Geometry: final body of the model. Coordinates: model frame, mm. Face numbers are marked on the shaded views. Give positions to 0.01 mm unless a question says otherwise; leave off trailing zeros. Order: outer loops, then holes, each group sorted by start corner. A loop starts at its lowest first (then second) coordinate and runs counter-clockwise, first axis right, second up. Notation, with made-up numbers: (-39.5, -10) - (2.5, -10) arc R30 cw to (2.5, 20) - close; hole circle Ø9 at (-24.75, 33.5). An arc over 180 degrees is marked (long way). Write item = value, one per line. Start each with the question number.
from build123d import *

# Parameters (mm, degrees)
BOSS_EXTRUDE1_DEPTH = 203.2


with BuildPart() as part:
    # Sketch1 → Boss-Extrude1 (new body)
    with BuildSketch(Plane.XY):
        Polygon((0, 0), (76.2, 0), (76.2, 19.05), (114.3, 19.05), (114.3, -12.7), (0, -12.7), align=None)
    boss_extrude1 = extrude(amount=-BOSS_EXTRUDE1_DEPTH)

    # Mirror1: Boss-Extrude1 across plane
    add(boss_extrude1.mirror(Plane(origin=(0, -12.7, -203.2), x_dir=(0, 0, 1), z_dir=(-1, 0, 0))))


solid = part.part
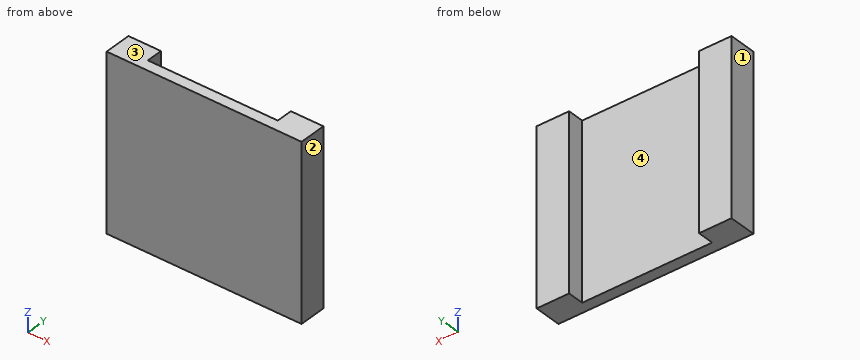
Q1. Section C-C, the plane x = -55. Return the cut outline in (y, z), then the cut area to 3 significant figures.
Q2. Section A-A, the plane y = 15. Return the cut outline in (x, z), then the cut area to 3 significant figures.
Q3. Pull-direction query (X, two-part tool) for the marked faces 1, 2, 3 and 4; classes: +X half, -X half, draft (parallel to the pull), parting line (faces both ways), or undercut.
Q4. Section B-B, the plane z = -126. Return the cut outline in (x, y), then the cut area to 3 significant figures.
Q5. Material intervals for line 1 along X through (y, z) = (1.5, -180); line 2 along Y through (x, z) = (-60, -102), sorted ascending. Write a range as from..to.
The answers:
q1.outline = (-12.7, -203.2) - (0, -203.2) - (0, 0) - (-12.7, 0) - close
q1.area = 2,580 mm²
q2.outline = (-114.3, -203.2) - (-76.2, -203.2) - (-76.2, 0) - (-114.3, 0) - close; (76.2, -203.2) - (114.3, -203.2) - (114.3, 0) - (76.2, 0) - close
q2.area = 15,500 mm²
q3.face_1 = -X half
q3.face_2 = +X half
q3.face_3 = draft
q3.face_4 = undercut
q4.outline = (-114.3, -12.7) - (114.3, -12.7) - (114.3, 19.05) - (76.2, 19.05) - (76.2, 0) - (-76.2, 0) - (-76.2, 19.05) - (-114.3, 19.05) - close
q4.area = 4,350 mm²
q5.line_1 = -114.3..-76.2, 76.2..114.3
q5.line_2 = -12.7..0
